from build123d import *

# Parameters (mm, degrees)
SKETCH1_R               = 3.175
SKETCH1_R_2             = 6.5
SKETCH1_R_3             = 1.1303
BOSS_EXTRUDE1_DEPTH     = 6.35
FILLET3_R               = 2
SKETCH4_R               = 11
BOSS_EXTRUDE2_DEPTH     = 7
CUT_EXTRUDE1_REACH      = 112.192
CUT_EXTRUDE1_END_RADIUS = 11
SKETCH2_R               = 1.1303


with BuildPart() as part:
    # Sketch1 → Boss-Extrude1 (new body)
    with BuildSketch(Plane.XY):
        with BuildLine():
            Line((-38.1, -12.7), (-38.1, 12.7))
            Line((-38.1, 12.7), (19.799208724, 12.7))
            Line((19.799208724, 12.7), (49.063216326, -5.044542368))
            ThreePointArc((49.063216326, -5.044542368), (63.185378941, -10.82071629), (66.044603929, -25.808194216))
            Line((66.044603929, -25.808194216), (62.155933896, -32.221324916))
            ThreePointArc((62.155933896, -32.221324916), (47.544550454, -36.615313538), (35.893587146, -26.763678338))
            Line((35.893587146, -26.763678338), (12.7, -12.7))
            Line((12.7, -12.7), (-38.1, -12.7))
        make_face()
        with Locations((-25.4, 0)):
            Circle(SKETCH1_R, mode=Mode.SUBTRACT)
        Circle(SKETCH1_R, mode=Mode.SUBTRACT)
        with Locations((50.8, -20.95)):
            Circle(SKETCH1_R_2, mode=Mode.SUBTRACT)
        with Locations((55.738610942, -12.805324011)):
            Circle(SKETCH1_R_3, mode=Mode.SUBTRACT)
        with Locations((45.861389058, -29.094675989)):
            Circle(SKETCH1_R_3, mode=Mode.SUBTRACT)
    extrude(amount=BOSS_EXTRUDE1_DEPTH)

    # Fillet3
    fillet3_edges = [part.edges().sort_by_distance(p)[0] for p in [
        (-38.1, -12.7, 3.175),
        (-38.1, 12.7, 3.175),
        (19.799208724, 12.7, 3.175),
        (12.7, -12.7, 3.175),
    ]]
    fillet(fillet3_edges, radius=FILLET3_R)

    # Sketch4 → Boss-Extrude2 (add)
    with BuildSketch(Plane.XY.offset(6.35)):
        with BuildLine():
            Line((66.044603929, -25.808194216), (62.155933896, -32.221324916))
            ThreePointArc((62.155933896, -32.221324916), (37.118654507, -12.654170595), (66.044603929, -25.808194216))
        make_face()
        with Locations((50.8, -20.95)):
            Circle(SKETCH4_R, mode=Mode.SUBTRACT)
    extrude(amount=BOSS_EXTRUDE2_DEPTH)

    # Cut-Extrude1: up to this cylinder (the profile starts outside it)
    cut_extrude1_end = Plane(origin=(50.8, -20.95, 9.85), z_dir=(0, 0, -1)) * Cylinder(CUT_EXTRUDE1_END_RADIUS, 247.384, mode=Mode.PRIVATE)
    # Sketch2 → Cut-Extrude1 (cut, up to the surface)
    with BuildSketch(Plane(origin=(59.73186838, -36.21905392, 0), x_dir=(0, 0, -1), z_dir=(0.8550840932924629, -0.5184893377864258, 0)), mode=Mode.PRIVATE) as cut_extrude1_sk1:
        with Locations(Location((-9.85, 8.425246605, 0), (0, 0, 90))):
            Circle(SKETCH2_R)
    cut_extrude1_tool1 = extrude(cut_extrude1_sk1.sketch, amount=-CUT_EXTRUDE1_REACH, mode=Mode.PRIVATE) - cut_extrude1_end
    add(cut_extrude1_tool1.solids().sort_by_distance((64.100269, -29.01476, 9.85))[0], mode=Mode.SUBTRACT)


solid = part.part
Geometry check sheet. Reference: the model listing, model coordinates, mm. A direction names the side the tool comes from. Round coordinates to 2 decimals unless told otherwise and drop trailing zeros. Order: outer loops, then holes, each group sorted by start corner. A loop starts at its lowest first (then second) coordinate and runs counter-clockwise, first axis right, second up. Notation, with made-up numbers: (72.25, 29) - (87.25, 29) arc R21 ccw to (87.25, 37) - close; hole circle Ø1 at (40, 62). An arc over 180 degrees is marked (long way). One line per question, with ' | ' between items. Start each with the question number.
(1) Sectioned sample at A-A on x = 0. Record the cut outline in (y, z) (3 decimals), and give its area (3 significant figures).
(2) Thickness scan on L1, parallel to X at y = -13, z = 6.25; L2, parallel to Y at x = 50.8, z = 3.5; L3, parallel to Y at x = 50.8, z = 8.5. Record the ranges inside material, lowest first. Write a range as [from, to].
(3) Access from +Z, -Z, +X, -X, +Y, -Y to the whole of each face (thin tool, end or side, straight path). Record for faces 1 (the cylindrical face through (48.42, -31.69, 9.8)), 2 (the flat face through (-12, -12.7, 3)), 3 (the flat face through (-38.1, 0, 3)).
(4) Release check for a two-part mould opening along Y. For faces 4 (the cylindrical face through (-37.53, -12.1, 3.22)), 5 (the flat face through (6, -2, 6.35)), 6 (the cylindrical face through (54.906, -12.041, 3.131)) record: released by +Y, released by -Y, zero draft, split by the parting line, or undercut.
(5) Sectioned sample at D-D on y = 0. Record the cut outline in (x, z) (3 decimals).
(6) Sectioned sample at C-C on z = 1.5. Record the cut outline in (x, y) (3 decimals), and give its area (3 significant figures).
(7) Sectioned sample at B-B on y = -22.5. Record the cut outline in (x, z), and give its area (3 significant figures).
(8) Depth check by flat-ended pin: pin 1 Ø12 at (x, y) = (-4.5, -12) entering from +Z; pin 2 Ø4 at (y, z) = (1, 6) entering from +X; pin 3 Ø6 at (y, z) = (0.5, 1.5) entering from +X. Enter the tip coordinate at first touch or a pass-through.
Conclusion:
1) outline: (-12.7, 0) - (-3.175, 0) - (-3.175, 6.35) - (-12.7, 6.35) - close; (3.175, 0) - (12.7, 0) - (12.7, 6.35) - (3.175, 6.35) - close | area: 121 mm2
2) L1: x = [13.19, 54.63], [56.85, 64.69] | L2: y = [-36.95, -27.45], [-14.45, -4.95] | L3: y = [-36.95, -31.95], [-9.95, -4.95]
3) face 1: +Z | face 2: +Z, -Z, -X, -Y | face 3: +Z, -Z, -X, +Y, -Y
4) face 4: released by -Y | face 5: zero draft | face 6: undercut
5) outline: (-38.1, 0) - (-28.575, 0) - (-28.575, 6.35) - (-38.1, 6.35) - close; (-22.225, 0) - (-3.175, 0) - (-3.175, 6.35) - (-22.225, 6.35) - close; (3.175, 0) - (40.744, 0) - (40.744, 6.35) - (3.175, 6.35) - close
6) outline: (-38.1, -10.7) arc R2 ccw to (-36.1, -12.7) - (12.141, -12.7) arc R2 cw to (13.178, -12.99) - (35.894, -26.764) arc R16 ccw to (62.156, -32.221) - (66.045, -25.808) arc R16 ccw to (49.063, -5.045) - (20.277, 12.41) arc R2 ccw to (19.24, 12.7) - (-36.1, 12.7) arc R2 ccw to (-38.1, 10.7) - close; hole circle Ø6.35 at (-25.4, 0); hole circle Ø6.35 at (0, 0); hole circle Ø13 at (50.8, -20.95); hole circle Ø2.261 at (45.861, -29.095); hole circle Ø2.261 at (55.739, -12.805) | area: 2,640 mm2
7) outline: (28.86, 0) - (44.49, 0) - (44.49, 6.35) - (39.91, 6.35) - (39.91, 13.35) - (34.88, 13.35) - (34.88, 6.35) - (28.86, 6.35) - close; (57.11, 0) - (66.72, 0) - (66.72, 13.35) - (61.69, 13.35) - (61.69, 6.35) - (57.11, 6.35) - close | area: 231 mm2
8) pin 1: stops at z = 6.35 | pin 2: stops at x = 42.39 | pin 3: stops at x = 44.87
